Source: CAD feature listing. Evaluate the final solid. Frame: model axes, mm. A direction names the side the tool comes from. Give positions to 0.01 mm unless a question says otherwise; leave off trailing zeros. Loops run counter-clockwise (first coordinate to the right, second up) from the corner with the lowest first, then second, coordinate; pieces in that order, holes last.
```python
from build123d import *

# Parameters (mm, degrees)
F2_DEPTH = 6
F1_R     = 10
F3_DEPTH = 6.001
F4_R     = 10
F5_DEPTH = 6.001


with BuildPart() as f2:
    # F0 (on Right) → F2 (new body)
    with BuildSketch(Plane.YZ):
        with BuildLine():
            Line((-54.603913, -329.447112), (196.299325, -329.447112))
            ThreePointArc((196.299325, -329.447112), (203.370393, -326.51818), (206.299325, -319.447112))
            Line((206.299325, -319.447112), (206.299325, -299.447112))
            ThreePointArc((206.299325, -299.447112), (203.370393, -292.376044), (196.299325, -289.447112))
            Line((196.299325, -289.447112), (56.466816, -289.447112))
            ThreePointArc((56.466816, -289.447112), (48.702245, -288.424887), (41.466816, -285.427874))
            Line((41.466816, -285.427874), (-9.578206, -255.957017))
            ThreePointArc((-9.578206, -255.957017), (-22.294592, -241.456758), (-23.555981, -222.211683))
            Line((-23.555981, -222.211683), (176.678757, 525.074533))
            ThreePointArc((176.678757, 525.074533), (179.67577, 532.309961), (184.443329, 538.523165))
            Line((184.443329, 538.523165), (233.612082, 587.691918))
            ThreePointArc((233.612082, 587.691918), (243.344782, 594.1951), (254.825285, 596.478714))
            Line((254.825285, 596.478714), (455.118371, 596.478714))
            ThreePointArc((455.118371, 596.478714), (462.189438, 599.407646), (465.118371, 606.478714))
            Line((465.118371, 606.478714), (465.118371, 626.478714))
            ThreePointArc((465.118371, 626.478714), (462.189438, 633.549782), (455.118371, 636.478714))
            Line((455.118371, 636.478714), (188.13818, 636.478714))
            ThreePointArc((188.13818, 636.478714), (169.875337, 630.279314), (159.160405, 614.243286))
            Line((159.160405, 614.243286), (-83.581688, -291.682541))
            ThreePointArc((-83.581688, -291.682541), (-78.404514, -317.709955), (-54.603913, -329.447112))
        make_face()
    extrude(amount=-F2_DEPTH)

    # F1 (on face) → F3 (cut, through all)
    with BuildSketch(Plane.YZ):
        with Locations((405.118371, 616.478714)):
            Circle(F1_R)
        with Locations((305.118371, 616.478714)):
            Circle(F1_R)
        with Locations((146.299325, -309.447112)):
            Circle(F1_R)
        with Locations((86.299325, -309.447112)):
            Circle(F1_R)
    extrude(amount=-F3_DEPTH, mode=Mode.SUBTRACT)

    # F4 (on face) → F5 (cut, through all)
    with BuildSketch(Plane.YZ):
        with Locations((208.13818, 616.478714)):
            Circle(F4_R)
        with Locations((208.459967, 591.478714)):
            Circle(F4_R)
        with Locations((5.944305, -288.012954)):
            Circle(F4_R)
        with Locations((-6.555695, -309.663589)):
            Circle(F4_R)
    extrude(amount=-F5_DEPTH, mode=Mode.SUBTRACT)


solid = f2.part
```
(1) Section B-B, the plane z = -90. Return the cut outline in (x, y).
A:
outline: (-6, -29.54) - (0, -29.54) - (0, 11.87) - (-6, 11.87) - close
(2) Mould query, pull axis Z, two halves, no side actions, for faces 3 (the flat face through (-2.96, 39.49, 167.62)), 4 (the flat face through (-3, 16.3, -270.9)), 5 (the flat face through (0, 67, 156)). Classes: pulls with the +Z half, pulls with the -Z half, needs draft (parallel to the pull), parting line crosses it, or undercut.
A:
face 3: pulls with the +Z half
face 4: undercut
face 5: needs draft
(3) Reachability of faces 1 (the flat face through (-2.96, 208.68, 562.76)), 2 (the cylindrical face through (-2.96, 145, -299.53)) from +Z, -Z, +X, -X, +Y, -Y: full face, straight path, thin tool, end or side. Return the list, or none.
A:
face 1: +X, -X, +Y
face 2: +X, -X
(4) Ray query, line 1 along Z through (x, y) = (-2.35, 205); line 2 along Z through (x, y) = (-4.25, 277.5); line 3 along Z through (x, y) = (-2.95, 401.5). Return the intervals inside material, ascending.
A:
line 1: z = -324.38 to -294.52, 559.08 to 582.1, 600.86 to 606.98, 625.97 to 636.48
line 2: z = 596.48 to 636.48
line 3: z = 596.48 to 607.16, 625.8 to 636.48
(5) First-contact query: pin 1 (1 mm diameter, centred on x = -4, y = 380, fed in from -Z); pin 2 (2 mm diameter, centred on x = -1, z = 127.5, fed in from -Y); pin 3 (3 mm diameter, centred on x = -4.5, z = 90, fed in from +Y). Flat tips, straight axial feed; report the tip coordinate or a pass-through.
A:
pin 1: stops at z = 596.48
pin 2: stops at y = 28.47
pin 3: stops at y = 60.5
(6) Section A-A, the plane x = -3.9. Count the separate pieces of the cut face and the enclosed holes in it, then the cut area to 3 significant figures.
A:
separate pieces: 1
enclosed holes: 8
area: 61,300 mm2
